The listing builds one solid part. Answer for the finished solid, in the listing's coordinates (mm). Face numbers are marked on the shaded views. A direction names the side the tool comes from. Coordinates: 2 decimals unless noted, no trailing zeros. Order: outer loops, then holes, each group sorted by start corner. A loop starts at its lowest first (then second) coordinate and runs counter-clockwise, first axis right, second up.
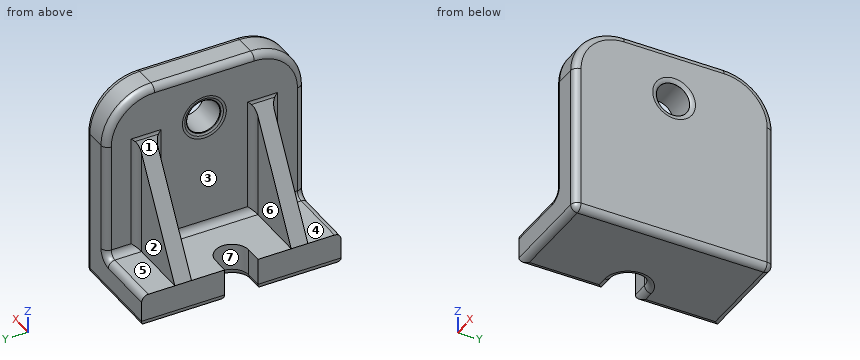
```python
from build123d import *

# Parameters (mm, degrees)
F1_DEPTH  = 76.2
F2_R      = 12.7
F3_DEPTH  = 76.201
F5_DEPTH  = 25.401
F6_R      = 38.1
F7_R      = 38.1
F10_DEPTH = 6.35
F11_SIZE  = 1.524
F12_SIZE  = 1.524
F13_R     = 5.08


# Not quite as in the source:
# - a length typed as a fraction of an inch, garbled in the dataset ("3 / 203.2 mm" for 3/8 in), is restored
# - a pattern or mirror of a feature is missing from the dataset's text; its kind, count and spacing are read off the source's solid


with BuildPart() as f1:
    # F0 (on Front) → F1 (new body, symmetric)
    with BuildSketch(Plane.XZ):
        Polygon((-76.2, 0), (0, 0), (0, 152.4), (-25.4, 152.4), (-25.4, 25.4), (-76.2, 25.4), align=None)
    extrude(amount=F1_DEPTH, both=True)

    # F2 (on face) → F3 (cut, through all)
    with BuildSketch(Plane.YZ):
        with Locations((0, 114.3)):
            Circle(F2_R)
    extrude(amount=-F3_DEPTH, mode=Mode.SUBTRACT)

    # F4 (on face) → F5 (cut, through all)
    with BuildSketch(Plane.XY.offset(25.4)):
        with BuildLine():
            ThreePointArc((-63.5, -12.7), (-50.8, 0), (-63.5, 12.7))
            Line((-63.5, 12.7), (-76.2, 12.7))
            Line((-76.2, 12.7), (-76.2, -12.7))
            Line((-76.2, -12.7), (-63.5, -12.7))
        make_face()
    extrude(amount=-F5_DEPTH, mode=Mode.SUBTRACT)

    # F6
    f6_edges = [f1.edges().sort_by_distance(p)[0] for p in [
        (-12.7, 76.2, 152.4),
    ]]
    fillet(f6_edges, radius=F6_R)

    # F7
    f7_edges = [f1.edges().sort_by_distance(p)[0] for p in [
        (-12.7, -76.2, 152.4),
    ]]
    fillet(f7_edges, radius=F7_R)

    # F9 (on offset) → F10 (join, symmetric)
    with BuildSketch(Plane.XZ.offset(44.45)):
        Polygon((-76.2, 25.4), (-25.4, 25.4), (-25.4, 114.3), align=None)
    f10 = extrude(amount=F10_DEPTH, both=True)

    # F10_copies: F10 across plane
    add(f10.mirror(Plane.ZX))

    # F11
    f11_edges = [f1.edges().sort_by_distance(p)[0] for p in [
        (0, -12.7, 114.3),
        (-12.7, 12.7, 114.3),
        (-25.4, -12.7, 114.3),
    ]]
    chamfer(f11_edges, length=F11_SIZE)

    # F12
    f12_edges = [f1.edges().sort_by_distance(p)[0] for p in [
        (-25.4, -14.224, 114.3),
    ]]
    chamfer(f12_edges, length=F12_SIZE)

    # F13
    f13_edges = [f1.edges().sort_by_distance(p)[0] for p in [
        (-25.4, -15.748, 114.3),
        (-25.4, -65.040768, 141.240768),
        (-25.4, -76.2, 69.85),
        (-25.4, -63.5, 25.4),
        (-25.4, -50.8, 69.85),
        (-25.4, -44.45, 114.3),
        (-25.4, -38.1, 69.85),
        (-25.4, 0, 25.4),
        (-25.4, 38.1, 69.85),
        (-25.4, 44.45, 114.3),
        (-25.4, 50.8, 69.85),
        (-25.4, 63.5, 25.4),
        (-25.4, 76.2, 69.85),
        (-25.4, 65.040768, 141.240768),
        (-25.4, 0, 152.4),
        (-12.7, -38.1, 152.4),
        (-12.7, 38.1, 152.4),
        (0, 0, 152.4),
        (0, 65.040768, 141.240768),
        (-12.7, 76.2, 114.3),
        (0, -65.040768, 141.240768),
        (-12.7, -76.2, 114.3),
        (0, -14.224, 114.3),
        (0, -76.2, 57.15),
        (0, 76.2, 57.15),
        (0, 0, 0),
        (-76.2, 44.45, 0),
        (-69.85, 12.7, 0),
        (-50.8, 0, 0),
        (-69.85, -12.7, 0),
        (-76.2, -44.45, 0),
        (-38.1, -76.2, 0),
        (-38.1, 76.2, 0),
        (-50.8, -76.2, 25.4),
        (-50.8, 76.2, 25.4),
    ]]
    fillet(f13_edges, radius=F13_R)


solid = f1.part
```
(1) Find section B-B (x = -67). Write down the section's boundary in (y, z).
(2) Find section C-C (z = 10). Write down the section's boundary in (x, y), and give its area (3 significant figures).
(3) Consider line 1 (Z direction, x = -17, y = 0); line 2 (Y direction, x = -13, z = 114); line 3 (Z direction, x = -39, y = 25.5). Determine where each line is inside the solid, lowest interval first.
(4) The mould has two halves that part along Y. Classify the marked faces 1, 2 and 3: released by +Y, released by -Y, zero draft, split by the parting line, or undercut.
(5) For the marked faces 4, 5, 6 and 7, determine the directions among +Z, -Z, +X, -X, +Y, -Y from which every point of the face is accessible in a straight line to the end or side of a thin tool.
(6) Find section A-A (y = 0). Write down the section's boundary in (x, z).
(7) Each of these flat-tipped pins is pushed along its axis until it touches: pin 1 Ø23 at (x, y) = (-50, 16.5) entering from +Z; pin 2 Ø13.5 at (x, z) = (-61.5, 54.5) entering from -Y; pin 3 Ø4 at (y, z) = (-43.5, 31.5) entering from -X. Where does it stop, or does it pass through?
(8) Find section D-D (x = -10). Write down the section's boundary in (y, z), and give its area (3 significant figures).
Findings below:
1. outline: (-76.2, 5.08) arc R5.08 ccw to (-71.12, 0) - (-17.78, 0) arc R5.08 ccw to (-12.7, 5.08) - (-12.7, 25.4) - (-38.1, 25.4) - (-38.1, 41.5) - (-50.8, 41.5) - (-50.8, 25.4) - (-71.12, 25.4) arc R5.08 ccw to (-76.2, 20.32) - close; (12.7, 5.08) arc R5.08 ccw to (17.78, 0) - (71.12, 0) arc R5.08 ccw to (76.2, 5.08) - (76.2, 20.32) arc R5.08 ccw to (71.12, 25.4) - (50.8, 25.4) - (50.8, 41.5) - (38.1, 41.5) - (38.1, 25.4) - (12.7, 25.4) - close
2. outline: (-76.2, -76.2) - (-5.08, -76.2) arc R5.08 ccw to (0, -71.12) - (0, 71.12) arc R5.08 ccw to (-5.08, 76.2) - (-76.2, 76.2) - (-76.2, 12.7) - (-63.5, 12.7) arc R12.7 cw to (-63.5, -12.7) - (-76.2, -12.7) - close
2. area: 11,000 mm2
3. line 1: z = 0 to 101.6, 127 to 152.4
3. line 2: y = -76.2 to -12.7, 12.7 to 76.2
3. line 3: z = 0 to 25.4
4. face 1: zero draft
4. face 2: released by +Y
4. face 3: undercut
5. face 4: +Z, -X, -Y
5. face 5: +Z, -X, +Y
5. face 6: +Z, -X
5. face 7: +Z, -Z, -X
6. outline: (-50.8, 5.08) arc R5.08 ccw to (-45.72, 0) - (-5.08, 0) arc R5.08 ccw to (0, 5.08) - (0, 97.97) arc R5.08 ccw to (-1.49, 101.56) - (-1.52, 101.6) - (-23.88, 101.6) - (-24.32, 101.15) - (-25.01, 99.49) arc R5.08 ccw to (-25.4, 97.54) - (-25.4, 30.48) arc R5.08 cw to (-30.48, 25.4) - (-50.8, 25.4) - close; (-25.4, 131.06) arc R5.08 ccw to (-25.01, 129.11) - (-24.32, 127.45) - (-23.88, 127) - (-1.52, 127) - (-1.49, 127.04) arc R5.08 ccw to (0, 130.63) - (0, 147.32) arc R5.08 ccw to (-5.08, 152.4) - (-20.32, 152.4) arc R5.08 ccw to (-25.4, 147.32) - close
7. pin 1: stops at z = 25.4
7. pin 2: stops at y = -50.8
7. pin 3: stops at x = -73.86
8. outline: (-76.2, 5.08) arc R5.08 ccw to (-71.12, 0) - (71.12, 0) arc R5.08 ccw to (76.2, 5.08) - (76.2, 114.3) arc R38.1 ccw to (38.1, 152.4) - (-38.1, 152.4) arc R38.1 ccw to (-76.2, 114.3) - close; hole circle Ø25.4 at (0, 114.3)
8. area: 22,100 mm2
